```python
from build123d import *

# Parameters (mm, degrees)
F0_R            = 6.35
F1_DEPTH        = 6.35
F3_D            = 1.27
F3_DEPTH        = 6.35
F3_CSINK_D      = 5.08
F3_CSINK_ANGLE  = 82
F3_TIP          = 0.3815464931
F3_COPIES_COUNT = 3


# Not quite as in the source:
# - a pattern or mirror of a feature is missing from the dataset's text; its kind, count and spacing are read off the source's solid


with BuildPart() as f1:
    # F0 (on Front) → F1 (new body)
    with BuildSketch(Plane.XZ):
        with BuildLine():
            ThreePointArc((37.338, -7.5818042708), (37.9090213538, -3.81), (38.1, 0))
            ThreePointArc((38.1, 0), (36.4813928036, 10.9871733904), (31.7630982094, 21.0408077825))
            ThreePointArc((31.7630982094, 21.0408077825), (29.4998029037, 24.1116492311), (26.9407683632, 26.9407683632))
            ThreePointArc((26.9407683632, 26.9407683632), (18.0271354281, 33.565345049), (7.5818042708, 37.338))
            ThreePointArc((7.5818042708, 37.338), (3.81, 37.9090213538), (0, 38.1))
            ThreePointArc((0, 38.1), (-10.9871733904, 36.4813928036), (-21.0408077825, 31.7630982094))
            ThreePointArc((-21.0408077825, 31.7630982094), (-24.1116492311, 29.4998029037), (-26.9407683632, 26.9407683632))
            ThreePointArc((-26.9407683632, 26.9407683632), (-33.565345049, 18.0271354281), (-37.338, 7.5818042708))
            ThreePointArc((-37.338, 7.5818042708), (-37.9090213538, 3.81), (-38.1, 0))
            ThreePointArc((-38.1, 0), (-36.4813928036, -10.9871733904), (-31.7630982094, -21.0408077825))
            ThreePointArc((-31.7630982094, -21.0408077825), (-29.4998029037, -24.1116492311), (-26.9407683632, -26.9407683632))
            ThreePointArc((-26.9407683632, -26.9407683632), (-18.0271354281, -33.565345049), (-7.5818042708, -37.338))
            ThreePointArc((-7.5818042708, -37.338), (-3.81, -37.9090213538), (0, -38.1))
            ThreePointArc((0, -38.1), (10.9871733904, -36.4813928036), (21.0408077825, -31.7630982094))
            ThreePointArc((21.0408077825, -31.7630982094), (24.1116492311, -29.4998029037), (26.9407683632, -26.9407683632))
            ThreePointArc((26.9407683632, -26.9407683632), (33.565345049, -18.0271354281), (37.338, -7.5818042708))
        make_face()
        Circle(F0_R, mode=Mode.SUBTRACT)
        with BuildLine():
            ThreePointArc((-26.9407683632, 26.9407683632), (-24.1116492311, 29.4998029037), (-21.0408077825, 31.7630982094))
            ThreePointArc((-21.0408077825, 31.7630982094), (-26.5592900173, 34.5512134403), (-32.3289220358, 32.3289220358))
            Line((-32.3289220358, 32.3289220358), (-26.9407683632, 26.9407683632))
        make_face()
        with BuildLine():
            ThreePointArc((0, 38.1), (3.81, 37.9090213538), (7.5818042708, 37.338))
            ThreePointArc((7.5818042708, 37.338), (5.6511432472, 43.2116513966), (0, 45.72))
            Line((0, 45.72), (0, 38.1))
        make_face()
        with BuildLine():
            ThreePointArc((26.9407683632, 26.9407683632), (29.4998029037, 24.1116492311), (31.7630982094, 21.0408077825))
            ThreePointArc((31.7630982094, 21.0408077825), (34.5512134403, 26.5592900173), (32.3289220358, 32.3289220358))
            Line((32.3289220358, 32.3289220358), (26.9407683632, 26.9407683632))
        make_face()
        with BuildLine():
            Line((45.72, 0), (38.1, 0))
            ThreePointArc((38.1, 0), (37.9090213538, -3.81), (37.338, -7.5818042708))
            ThreePointArc((37.338, -7.5818042708), (43.2116513966, -5.6511432472), (45.72, 0))
        make_face()
        with BuildLine():
            Line((32.3289220358, -32.3289220358), (26.9407683632, -26.9407683632))
            ThreePointArc((26.9407683632, -26.9407683632), (24.1116492311, -29.4998029037), (21.0408077825, -31.7630982094))
            ThreePointArc((21.0408077825, -31.7630982094), (26.5592900173, -34.5512134403), (32.3289220358, -32.3289220358))
        make_face()
        with BuildLine():
            Line((0, -45.72), (0, -38.1))
            ThreePointArc((0, -38.1), (-3.81, -37.9090213538), (-7.5818042708, -37.338))
            ThreePointArc((-7.5818042708, -37.338), (-5.6511432472, -43.2116513966), (0, -45.72))
        make_face()
        with BuildLine():
            Line((-32.3289220358, -32.3289220358), (-26.9407683632, -26.9407683632))
            ThreePointArc((-26.9407683632, -26.9407683632), (-29.4998029037, -24.1116492311), (-31.7630982094, -21.0408077825))
            ThreePointArc((-31.7630982094, -21.0408077825), (-34.5512134403, -26.5592900173), (-32.3289220358, -32.3289220358))
        make_face()
        with BuildLine():
            ThreePointArc((-38.1, 0), (-37.9090213538, 3.81), (-37.338, 7.5818042708))
            ThreePointArc((-37.338, 7.5818042708), (-43.2116513966, 5.6511432472), (-45.72, 0))
            Line((-45.72, 0), (-38.1, 0))
        make_face()
    extrude(amount=F1_DEPTH)

    # F3
    with Locations(Plane.XZ.offset(6.35)):
        with Locations((0, 17.78)):
            f3 = CounterSinkHole(F3_D / 2, F3_CSINK_D / 2, depth=F3_DEPTH, counter_sink_angle=F3_CSINK_ANGLE)
            with Locations((0, 0, -(F3_DEPTH + F3_TIP / 2))):  # 118° drill point
                Cone(0, F3_D / 2, F3_TIP, mode=Mode.SUBTRACT)

    # F3_copies: F3 ×3 about axis
    f3_copies_axis = Axis((0, 0, 0), (0, 1, 0))
    for i in range(1, F3_COPIES_COUNT):
        add(f3.rotate(f3_copies_axis, i * 360 / F3_COPIES_COUNT), mode=Mode.SUBTRACT)


solid = f1.part
```
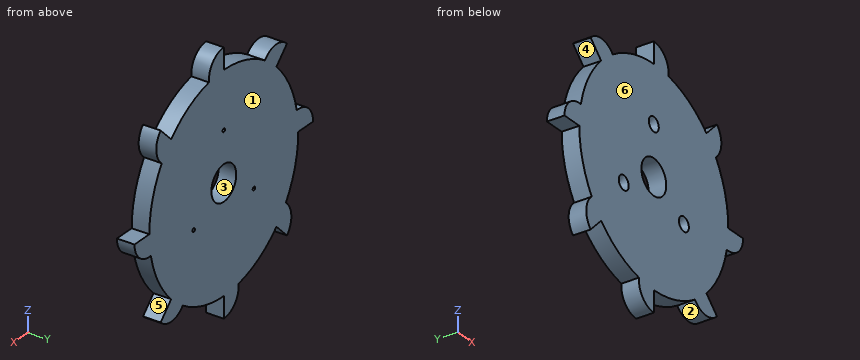
Can you work these out from the model? Positions are in its coordinate system, mm. Face numbers are marked on the shaded views. A direction names the side the tool comes from. Coordinates: 2 decimals unless noted, no trailing zeros. Write each loop counter-clockwise with the first axis right and the second up, starting at its lowest first coordinate (ties: lowest second). Pieces come first, ordered by that corner, then holes. Notation, with made-up numbers: (67.25, -22.5) - (74.25, -22.5) arc R30 ccw to (74.25, 2.5) - close; hole circle Ø2 at (81.25, 11). An arc over 180 degrees is marked (long way). Return JSON: item names as keys, results as strings.
Q1. If we section it at B-B (z = 40.5): Please give me the cut outline in (x, y).
Computed values:
{"outline": "(0, -6.35) - (7.23, -6.35) - (7.23, 0) - (0, 0) - close"}
Q2. I'm going to push flat-ended pins straight in: pin 1 Ø1.9 at (x, y) = (41, -2) entering from +Z; pin 2 Ø1.9 at (y, z) = (-4, -43.5) entering from +X; pin 3 Ø7.5 at (x, z) = (0, 0) entering from +Y; pin 4 Ø1.9 at (x, y) = (-41, -2.5) entering from -Z. Where does each tip first touch, or does it pass through?
Computed values:
{"pin 1": "stops at z = 0", "pin 2": "stops at x = 0", "pin 3": "passes through", "pin 4": "stops at z = 0"}
Q3. Please list where these lines run through material, in increasing order: L1, parallel to X at y = -1.45, z = -8.89; L2, parallel to X at y = -3, z = 3; L3, parallel to Z at x = -31, y = -2.25. Write a range as from..to.
Computed values:
{"L1": "x = -37.05..-16.03, -14.76..14.76, 16.03..37.05", "L2": "x = -45.1..-5.6, 5.6..37.98", "L3": "z = -31..22.15, 31..33.39"}
Q4. If we section it at A-A (y = -5.25): Please give me the cut outline in (x, z).
Computed values:
{"outline": "(-45.72, 0) - (-38.1, 0) arc R38.1 ccw to (-31.76, -21.04) arc R7.62 ccw to (-32.33, -32.33) - (-26.94, -26.94) arc R38.1 ccw to (-7.58, -37.34) arc R7.62 ccw to (0, -45.72) - (0, -38.1) arc R38.1 ccw to (21.04, -31.76) arc R7.62 ccw to (32.33, -32.33) - (26.94, -26.94) arc R38.1 ccw to (37.34, -7.58) arc R7.62 ccw to (45.72, 0) - (38.1, 0) arc R38.1 ccw to (31.76, 21.04) arc R7.62 ccw to (32.33, 32.33) - (26.94, 26.94) arc R38.1 ccw to (7.58, 37.34) arc R7.62 ccw to (0, 45.72) - (0, 38.1) arc R38.1 ccw to (-21.04, 31.76) arc R7.62 ccw to (-32.33, 32.33) - (-26.94, 26.94) arc R38.1 ccw to (-37.34, 7.58) arc R7.62 ccw to start; hole circle Ø3.17 at (-15.4, -8.89); hole circle Ø12.7 at (0, 0); hole circle Ø3.17 at (0, 17.78); hole circle Ø3.17 at (15.4, -8.89)"}
Q5. Thinking about a two-plate mould opening in Z: for the marked faces 1, 2 and 3, which applies, +Z half, -Z half, draft (parallel to the pull), parting line (faces both ways), or undercut?
Computed values:
{"face 1": "draft", "face 2": "-Z half", "face 3": "undercut"}
Q6. On a 3-axis mill with a long thin cutter (end or side, diameter ignored), from which of +Z, -Z, +X, -X, +Y, -Y can I reach the whole of each face in a straight line? I mean the marked faces 4, 5 and 6. Say none if no direction works.
Computed values:
{"face 4": "-X, +Y, -Y", "face 5": "+X, +Y, -Y", "face 6": "+Z, -Z, +X, -X, -Y"}
Q7. If we section it at C-C (x = -9.5): Please give me the cut outline in (y, z).
Computed values:
{"outline": "(-6.35, -36.9) - (0, -36.9) - (0, 36.9) - (-6.35, 36.9) - close"}
